from build123d import *

# Parameters (mm, degrees)
SKETCH_2_W                  = 93.1
SKETCH_2_H                  = 10
EXTRUDE_1_DEPTH             = 3.5
SKETCH_4_W                  = 93.1
SKETCH_4_H                  = 6.5
EXTRUDE_2_DEPTH             = 1.1
SKETCH_5_W                  = 93.1
SKETCH_5_H                  = 10
EXTRUDE_3_DEPTH             = 2
CUT_EXTRUDE_1_DEPTH         = 94.867832616
SKETCH_7_W                  = 83.1
SKETCH_7_H                  = 1.1
EXTRUDE_4_DEPTH             = 3.5
CHAMFER_1_SIZE              = 0.4
CUT_EXTRUDE_2_REACH         = 95.868
SKETCH_8_R                  = 150
SKETCH_9_W                  = 93.1
SKETCH_9_H                  = 2
EXTRUDE_5_DEPTH             = 5
EXTRUDE_5_DIRECTION_2_REACH = 95.868
SKETCH_10_W                 = 93.1
SKETCH_10_H                 = 7.621023553
EXTRUDE_6_DEPTH             = 2
SKETCH_11_W                 = 1
SKETCH_11_H                 = 7.621023553
CUT_EXTRUDE_3_DEPTH         = 1


with BuildPart() as part:
    # 草图2 → 凸台-拉伸1 (new body)
    with BuildSketch(Plane(origin=(0, 0, 0), x_dir=(1, 0, 0), z_dir=(0, 1, 0))):
        with Locations((46.55, 5)):
            Rectangle(SKETCH_2_W, SKETCH_2_H)
    extrude(amount=EXTRUDE_1_DEPTH)

    # 草图4 → 凸台-拉伸2 (add)
    with BuildSketch(Plane(origin=(0, 3.5, 0), x_dir=(1, 0, 0), z_dir=(0, 1, 0))):
        with Locations((46.55, 6.75)):
            Rectangle(SKETCH_4_W, SKETCH_4_H)
    extrude(amount=EXTRUDE_2_DEPTH)

    # 草图5 → 凸台-拉伸3 (add)
    with BuildSketch(Plane(origin=(0, 4.6, 0), x_dir=(1, 0, 0), z_dir=(0, 1, 0))):
        with Locations((46.55, 5)):
            Rectangle(SKETCH_5_W, SKETCH_5_H)
    extrude(amount=EXTRUDE_3_DEPTH)

    # 草图6 → 切除-拉伸1 (cut, through all)
    with BuildSketch(Plane.ZY):
        Polygon((-10, 0), (-6.189488223, 6.6), (-10, 6.6), align=None)
    extrude(amount=-CUT_EXTRUDE_1_DEPTH, mode=Mode.SUBTRACT)

    # 草图7 → 凸台-拉伸4 (add)
    with BuildSketch(Plane.XY.offset(-3.5)):
        with Locations((46.55, 4.05)):
            Rectangle(SKETCH_7_W, SKETCH_7_H)
    extrude(amount=EXTRUDE_4_DEPTH)

    # 倒角1
    chamfer_1_edges = [part.edges().sort_by_distance(p)[0] for p in [
        (90.6, 3.5, 0),
        (2.5, 3.5, 0),
    ]]
    chamfer(chamfer_1_edges, length=CHAMFER_1_SIZE)

    # 草图8 → 切除-拉伸2 (cut, up to next)
    with BuildSketch(Plane.XZ, mode=Mode.PRIVATE) as cut_extrude_2_sk1:
        with Locations((46.55, 147)):
            Circle(SKETCH_8_R)
    cut_extrude_2_tool1 = extrude(cut_extrude_2_sk1.sketch, amount=-CUT_EXTRUDE_2_REACH, mode=Mode.PRIVATE) & part.part
    add(cut_extrude_2_tool1.solids().sort_by_distance((46.55, 0, 147))[0], mode=Mode.SUBTRACT)

    # 草图9 → 凸台-拉伸5 (add)
    with BuildSketch(Plane.XY):
        with Locations((46.55, 5.6)):
            Rectangle(SKETCH_9_W, SKETCH_9_H)
    extrude(amount=EXTRUDE_5_DEPTH)

    # 草图9 → 凸台-拉伸5 direction 2 (add, up to next)
    with BuildSketch(Plane.XY, mode=Mode.PRIVATE) as extrude_5_direction_2_sk1:
        with Locations((46.55, 5.6)):
            Rectangle(SKETCH_9_W, SKETCH_9_H)
    extrude_5_direction_2_tool1 = extrude(extrude_5_direction_2_sk1.sketch, amount=-EXTRUDE_5_DIRECTION_2_REACH, mode=Mode.PRIVATE) - part.part
    add(extrude_5_direction_2_tool1.solids().sort_by_distance((46.55, 5.6, 0))[0])

    # 草图10 → 凸台-拉伸6 (add, along a direction that is not the sketch's normal)
    with BuildSketch(Plane(origin=(0, 4.330127019, -7.5), x_dir=(-1, 0, 0), z_dir=(0, 0.4999999999999947, -0.8660254037844417))):
        with Locations((-46.55, -1.189488223)):
            Rectangle(SKETCH_10_W, SKETCH_10_H)
    extrude(amount=EXTRUDE_6_DEPTH, dir=(0, 0, -1))

    # 草图11 → 切除-拉伸3 (cut, along a direction that is not the sketch's normal)
    with BuildSketch(Plane(origin=(0, 5.196152423, -9), x_dir=(-1, 0, 0), z_dir=(0, 0.49999999999999484, -0.8660254037844418))):
        with Locations((-46.05, -2.189488223)):
            Rectangle(SKETCH_11_W, SKETCH_11_H)
        with Locations((-36.05, -2.189488223)):
            Rectangle(SKETCH_11_W, SKETCH_11_H)
    extrude(amount=-CUT_EXTRUDE_3_DEPTH, dir=(0, 0, -1), mode=Mode.SUBTRACT)


solid = part.part
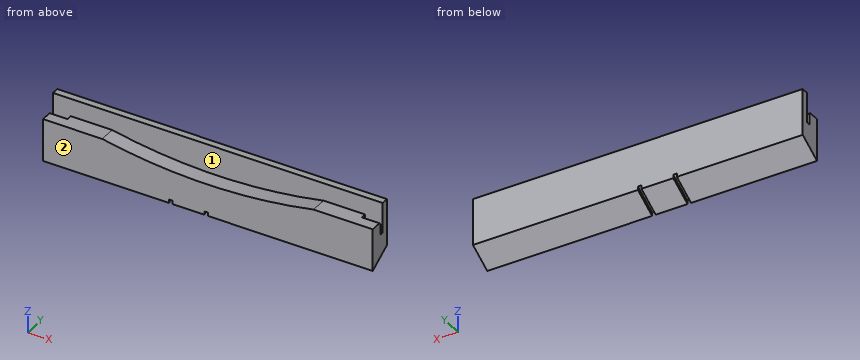
Geometry: final body of the model. Coordinates: model frame, mm. Face numbers are marked on the shaded views. Round coordinates to 2 decimals unless told otherwise and drop trailing zeros. Loops run counter-clockwise (first coordinate to the right, second up) from the corner with the lowest first, then second, coordinate; pieces in that order, holes last.
Q1. Section D-D on x = 56. Return loops of the section in (y, z).
Q2. Section A-A on y = 1.5. Return loops of the section in (x, z).
Q3. Material intervals for L1, parallel to X at y = 3, z = -9.75; L2, parallel to Y at x = 12.5, z = 1; L3, parallel to Z at x = 22, y = 1.5, sorted ascending.
Q4. Pin query (flat end, axial travel): P1, Ø0.9, axis at x = 1.5, y = 4, coming from the +Z side; P2, Ø2, axis at y = 1.5, z = 2.5, coming from the -X side; P3, Ø1.4, axis at x = 84, y = 1.5, coming from the +Z side. Return the tip coordinate at first contact, or that it passes through.
Q5. Pull-direction query (X, two-part tool) for the marked faces 1 and 2; classes: released by +X, released by -X, zero draft, split by the parting line, or undercut.
Q6. Section B-B on x = 82.5. Return loops of the section in (y, z).
Evaluation:
1. outline: (0, -12) - (6.6, -8.19) - (6.6, 5) - (4.6, 5) - (4.6, -2.7) - (0, -2.7) - close
2. outline: (0, -11.13) - (35.55, -11.13) - (35.55, -10.13) - (36.55, -10.13) - (36.55, -11.13) - (45.55, -11.13) - (45.55, -10.13) - (46.55, -10.13) - (46.55, -11.13) - (93.1, -11.13) - (93.1, 0) - (76.4, 0) arc R150 cw to (16.7, 0) - (0, 0) - close
3. L1: x = 0 to 35.55, 36.55 to 45.55, 46.55 to 93.1
3. L2: y = 4.6 to 6.6
3. L3: z = -11.13 to -0.98
4. P1: stops at z = -3.5
4. P2: passes through
4. P3: stops at z = 0
5. face 1: undercut
5. face 2: zero draft
6. outline: (0, -12) - (6.6, -8.19) - (6.6, 5) - (4.6, 5) - (4.6, 0) - (0, 0) - close
